Could you check a few things on this drawing? It's one solid part, dimensions in mm from its lowest x, y, z. A direction names the side the tool comes from. Coordinates: 2 decimals unless noted, no trailing zeros. Write each loop counter-clockwise with the first axis right and the second up, starting at its lowest first coordinate (ties: lowest second). Pieces come first, ordered by that corner, then holes. Notation, with made-up numbers: M -13,16.25 L 4,16.25 A15 ccw 4,32.25 Z; hole C -4,41 d2. An arc over 180 degrees is marked long. Use a Markdown table: item, result.
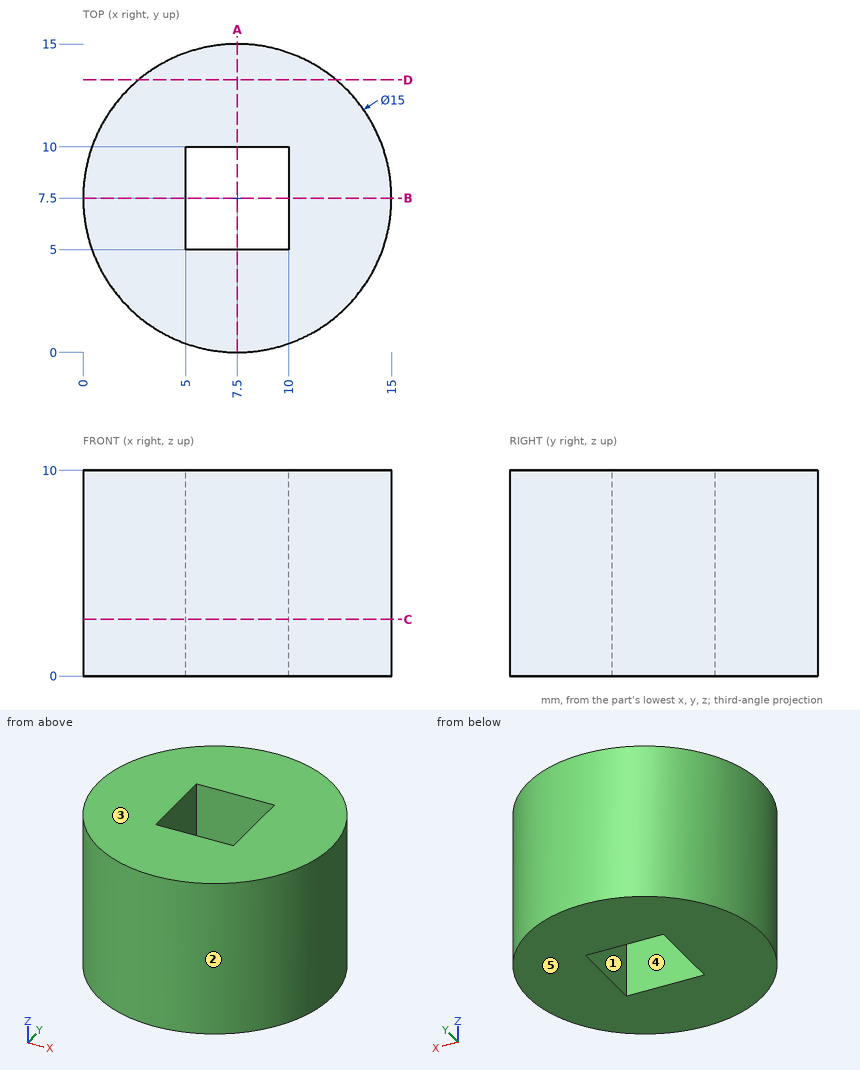
1. We'd pull the mould along Y, two halves only. Please class the marked faces 1, 2 and 3: +Y half, -Y half, draft (parallel to the pull), parting line (faces both ways), or undercut.
Answers follow:
| item | result |
|---|---|
| face 1 | undercut |
| face 2 | parting line |
| face 3 | draft |
2. I need wall thicknesses on probe 1 along Y at (x, z) = (8.75, 4.75); probe 2 along X at (y, z) = (7, 1.25); probe 3 along X at (y, z) = (9, 7.25). Which ranges of each line are inside material? Lowest first, please.
Answers follow:
| item | result |
|---|---|
| probe 1 | y = 0.1 to 5, 10 to 14.9 |
| probe 2 | x = 0.02 to 5, 10 to 14.98 |
| probe 3 | x = 0.15 to 5, 10 to 14.85 |
3. Will these pins go through, and if not, where does the flat tip stop? pin 1 Ø2 at (y, z) = (3.5, 2) entering from +X; pin 2 Ø2 at (x, z) = (2.5, 6.5) entering from -Y; pin 3 Ø3 at (y, z) = (5.5, 3.5) entering from -X.
Answers follow:
| item | result |
|---|---|
| pin 1 | stops at x = 14.37 |
| pin 2 | stops at y = 1.16 |
| pin 3 | stops at x = 0.02 |
4. Suppose I cut it at C-C on z = 2.75. Write out the boundary of the cut face in (x, y), and give its area (3 significant figures).
Answers follow:
| item | result |
|---|---|
| outline | C 7.5,7.5 d15; hole M 5,5 L 10,5 L 10,10 L 5,10 Z |
| area | 152 mm2 |
5. Suppose I cut it at D-D on y = 13.25. Write out the boundary of the cut face in (x, z).
Answers follow:
| item | result |
|---|---|
| outline | M 2.68,0 L 12.32,0 L 12.32,10 L 2.68,10 Z |
6. Suppose I cut it at A-A on x = 7.5. Write out the boundary of the cut face in (y, z).
Answers follow:
| item | result |
|---|---|
| outline | M 0,0 L 5,0 L 5,10 L 0,10 Z; M 10,0 L 15,0 L 15,10 L 10,10 Z |
7. Which directions (+Z, -Z, +X, -X, +Y, -Y) give clear straight access to the entire face, cutting with the end or side of a thin tool? Please do the marked faces 4 and 5.
Answers follow:
| item | result |
|---|---|
| face 4 | +Z, -Z |
| face 5 | -Z, +X, -X, +Y, -Y |
